Input: part model. Units: mm. Frame: model coordinates. A direction names the side the tool comes from. Round coordinates to 2 decimals unless told otherwise and drop trailing zeros. Order: outer loops, then holes, each group sorted by start corner. A loop starts at its lowest first (then second) coordinate and runs counter-clockwise, first axis right, second up. Notation, with made-up numbers: (45.25, 65.25) - (94.25, 65.25) arc R19 cw to (94.25, 83.25) - close; hole circle Ø10 at (15, 47). An arc over 180 degrees is marked (long way). One line per item, written item: value. Start each with the question number.
from build123d import *

# Parameters (mm, degrees)
F1_DEPTH  = 50
F2_R      = 5.5
F3_DEPTH  = 22.5
F5_W      = 19.5
F5_H      = 50
F6_DEPTH  = 90
F7_R      = 4
F8_DEPTH  = 50.001
F9_R      = 2.5
F10_DEPTH = 50
F11_R     = 4
F12_DEPTH = 40


with BuildPart() as f1:
    # F0 (on Top) → F1 (new body)
    with BuildSketch(Plane.XY):
        with BuildLine():
            Line((0, -21.5), (63.984373, -21.5))
            ThreePointArc((63.984373, -21.5), (67.5, 0), (63.984373, 21.5))
            Line((63.984373, 21.5), (0, 21.5))
            Line((0, 21.5), (-63.984373, 21.5))
            ThreePointArc((-63.984373, 21.5), (-67.5, 0), (-63.984373, -21.5))
            Line((-63.984373, -21.5), (0, -21.5))
        make_face()
    extrude(amount=F1_DEPTH)


with BuildPart() as f3:
    # F2 (on Front) → F3 (new body, symmetric)
    with BuildSketch(Plane.XZ):
        with BuildLine():
            Line((-67.518182, 0), (67.335986, 0))
            ThreePointArc((67.335986, 0), (-0.091098, 50.000059), (-67.518182, 0))
        make_face()
        with Locations((0, 40)):
            Circle(F2_R, mode=Mode.SUBTRACT)
    extrude(amount=F3_DEPTH, both=True)


with BuildPart() as f1_1:
    add(f1.part)

    # F4: intersect F3
    add(f3.part, mode=Mode.INTERSECT)

    # F5 (on Right) → F6 (cut, symmetric)
    with BuildSketch(Plane.YZ):
        with Locations((-9.75, 27)):
            Rectangle(F5_W, F5_H)
        with Locations((9.75, 27)):
            Rectangle(F5_W, F5_H)
    extrude(amount=F6_DEPTH, both=True, mode=Mode.SUBTRACT)

    # F7 (on Top) → F8 (cut, through all)
    with BuildSketch(Plane.XY):
        with Locations((57, 0)):
            Circle(F7_R)
        with Locations((-57, 0)):
            Circle(F7_R)
    extrude(amount=F8_DEPTH, mode=Mode.SUBTRACT)

    # F9 (on Front) → F10 (cut)
    with BuildSketch(Plane.XZ):
        with Locations((-47.5, 24)):
            Circle(F9_R)
        with Locations((47.5, 24)):
            Circle(F9_R)
    extrude(amount=-F10_DEPTH, mode=Mode.SUBTRACT)

    # F11 (on Front) → F12 (cut)
    with BuildSketch(Plane.XZ):
        with Locations((47.5, 24)):
            Circle(F11_R)
        with Locations((-47.5, 24)):
            Circle(F11_R)
    extrude(amount=F12_DEPTH, mode=Mode.SUBTRACT)


solid = f1_1.part
1. Section D-D (z = 10.5). Return the cut outline in (x, y), then the cut area to 3 significant figures.
2. Set-up query: faces 5 (the face through (39.158, 20.486, 38.057)), 6 (the face through (1, 0, 2)), 7 (the face through (-50.45, -20.49, 26.7)). Return all of +Z, -Z, +X, -X, +Y, -Y with unobstructed straight access to the full face (end or side cutting, diameter ignored); none if empty.
3. Line query: line 1 (Z direction, x = 0, y = -20); line 2 (Y direction, x = -19.5, z = 39.5); line 3 (X direction, y = 0, z = 1.3). Output: solid intervals per line, ascending. Write a range as from..to.
4. Section A-A (y = 0). Return the cut outline in (x, z), then the cut area to 3 significant figures.
5. Pull-direction query (Z, two-part tool) for faces 1 (the face through (-0.716, -20.486, 45.453)), 2 (the face through (1, 21.5, 19)), 3 (the face through (-1, 0, 0)), 4 (the face through (-46, 20, 26)); classes: released by +Z, released by -Z, zero draft, split by the parting line, or undercut.
6. Pin query (flat end, axial travel): pin 1 (5 mm diameter, centred on x = -48, y = -12, fed in from +Z); pin 2 (4 mm diameter, centred on x = -47.5, z = 24, fed in from +Y). Return the tip coordinate at first contact, or that it passes through.
7. Section C-C (x = -47.5). Return the cut outline in (y, z).
8. Section B-B (z = 42.5). Return the cut outline in (x, y).
Solved:
1. outline: (-63.39, -21.5) - (63.21, -21.5) - (63.21, -19.5) - (-63.39, -19.5) - close; (-63.39, 19.5) - (63.21, 19.5) - (63.21, 21.5) - (-63.39, 21.5) - close
1. area: 506 mm²
2. face 5: +Z, +X, +Y, -Y
2. face 6: +Z, +X, -X
2. face 7: -Y
3. line 1: z = 0..34.5, 45.5..50
3. line 2: y = -21.5..-19.5, 19.5..21.5
3. line 3: x = -67.11..-61, -53..53, 61..66.93
4. outline: (-67.5, 0) - (-61, 0) - (-61, 2) - (-66.88, 2) arc R70.46 ccw to (-67.5, 0.06) - close; (-53, 0) - (53, 0) - (53, 2) - (-53, 2) - close; (61, 0) - (67.34, 0) arc R70.46 ccw to (66.7, 2) - (61, 2) - close
4. area: 236 mm²
5. face 1: undercut
5. face 2: zero draft
5. face 3: released by -Z
5. face 4: undercut
6. pin 1: stops at z = 2
6. pin 2: passes through
7. outline: (-21.5, 0) - (21.5, 0) - (21.5, 21.5) - (19.5, 21.5) - (19.5, 2) - (-19.5, 2) - (-19.5, 20) - (-21.5, 20) - close; (-21.5, 28) - (-19.5, 28) - (-19.5, 31.67) - (-21.5, 31.67) - close; (19.5, 26.5) - (21.5, 26.5) - (21.5, 31.67) - (19.5, 31.67) - close
8. outline: (-31.73, -21.5) - (-4.9, -21.5) - (-4.9, -19.5) - (-31.73, -19.5) - close; (-31.73, 19.5) - (-4.9, 19.5) - (-4.9, 21.5) - (-31.73, 21.5) - close; (4.9, -21.5) - (31.54, -21.5) - (31.54, -19.5) - (4.9, -19.5) - close; (4.9, 19.5) - (31.54, 19.5) - (31.54, 21.5) - (4.9, 21.5) - close
